```python
from build123d import *

# Parameters (mm, degrees)
F0_W     = 100
F0_H     = 100
F1_DEPTH = 100
F2_R     = 10
F3_R     = 15
F4_DEPTH = 100.001
F5_R     = 6
F6_DEPTH = 36.2532730151
F7_W     = 150
F7_H     = 100
F8_DEPTH = 25
F9_R     = 5
F11_D    = 10


with BuildPart() as f1:
    # F0 (on Front) → F1 (new body)
    with BuildSketch(Plane.XZ):
        Rectangle(F0_W, F0_H)
    extrude(amount=F1_DEPTH)

    # F2
    f2_edges = [f1.edges().sort_by_distance(p)[0] for p in [
        (50, -100, 0),
        (-50, -100, 0),
    ]]
    fillet(f2_edges, radius=F2_R)

    # F3 (on face) → F4 (cut, through all)
    with BuildSketch(Plane.XY.offset(50)):
        with Locations((0, -50)):
            Circle(F3_R)
    extrude(amount=-F4_DEPTH, mode=Mode.SUBTRACT)

    # F5 (on face) → F6 (cut, through all)
    with BuildSketch(Plane.XZ.offset(100)):
        Circle(F5_R)
    extrude(amount=-F6_DEPTH, mode=Mode.SUBTRACT)

    # F7 (on Front) → F8 (join)
    with BuildSketch(Plane.XZ):
        Rectangle(F7_W, F7_H)
    extrude(amount=-F8_DEPTH)

    # F9
    f9_edges = [f1.edges().sort_by_distance(p)[0] for p in [
        (50, 0, 0),
        (-50, 0, 0),
    ]]
    fillet(f9_edges, radius=F9_R)

    # F11 (through all)
    with Locations(Plane.XZ):
        with Locations((-65, 25), (-65, -25), (65, 25), (65, -25)):
            Hole(F11_D / 2)


solid = f1.part
```
Input: part model. Units: mm. Frame: model coordinates. A direction names the side the tool comes from. Give positions to 0.01 mm unless a question says otherwise; leave off trailing zeros. Order: outer loops, then holes, each group sorted by start corner. A loop starts at its lowest first (then second) coordinate and runs counter-clockwise, first axis right, second up. Notation, with made-up numbers: (27.5, 63) - (72.5, 63) arc R11 ccw to (72.5, 70) - close; hole circle Ø6 at (77.25, 33). An arc over 180 degrees is marked (long way). One line per item, written item: value.
1. Cut plane A-A, the plane z = 25. Output: boundary loops of the cut face in (x, y), and give its area (3 significant figures).
Determined:
outline: (-75, 0) - (-70, 0) - (-70, 25) - (-75, 25) - close; (-60, 0) - (-55, 0) arc R5 cw to (-50, -5) - (-50, -90) arc R10 ccw to (-40, -100) - (40, -100) arc R10 ccw to (50, -90) - (50, -5) arc R5 cw to (55, 0) - (60, 0) - (60, 25) - (-60, 25) - close; (70, 0) - (75, 0) - (75, 25) - (70, 25) - close; hole circle Ø30 at (0, -50)
area: 12,500 mm2
2. Cut plane D-D, the plane z = 0. Output: boundary loops of the cut face in (x, y), and give its area (3 significant figures).
Determined:
outline: (-75, 0) - (-55, 0) arc R5 cw to (-50, -5) - (-50, -90) arc R10 ccw to (-40, -100) - (-6, -100) - (-6, -63.75) arc R15 cw (long way) to (6, -63.75) - (6, -100) - (40, -100) arc R10 ccw to (50, -90) - (50, -5) arc R5 cw to (55, 0) - (75, 0) - (75, 25) - (-75, 25) - close
area: 12,600 mm2
3. Pin query (flat end, axial travel): pin 1 Ø6 at (y, z) = (-27, 1.5) entering from +X; pin 2 Ø12 at (x, z) = (48, -5) entering from -Y; pin 3 Ø10 at (x, z) = (-62.5, 24) entering from -Y; pin 4 Ø10 at (x, z) = (42.5, -29) entering from -Y. Return the tip coordinate at first contact, or that it passes through.
Determined:
pin 1: x = 50
pin 2: y = -99.8
pin 3: y = 0
pin 4: y = -100
4. Line query: probe 1 along Z at (x, y) = (-65, 15.5); probe 2 along X at (y, z) = (-82, 0); probe 3 along X at (y, z) = (-85, 11). Output: solid intervals per line, ascending.
Determined:
probe 1: -50 to -30, -20 to 20, 30 to 50
probe 2: -50 to -6, 6 to 50
probe 3: -50 to 50
5. Cut plane C-C, the plane y = -59. Output: boundary loops of the cut face in (x, z), and give its area (3 significant figures).
Determined:
outline: (-50, -50) - (-12, -50) - (-12, 50) - (-50, 50) - close; (12, -50) - (50, -50) - (50, 50) - (12, 50) - close
area: 7,600 mm2
6. Cut plane B-B, the plane x = -65. Output: boundary loops of the cut face in (y, z), and give its area (3 significant figures).
Determined:
outline: (0, -50) - (25, -50) - (25, -30) - (0, -30) - close; (0, -20) - (25, -20) - (25, 20) - (0, 20) - close; (0, 30) - (25, 30) - (25, 50) - (0, 50) - close
area: 2,000 mm2
7. Reachability of faces 4 (the face through (-65, 0, 1)), 5 (the face through (66.08, 12.68, 20.12)), 6 (the face through (65, 0, 1)) from +Z, -Z, +X, -X, +Y, -Y: full face, straight path, thin tool, end or side. Return the list, or none.
Determined:
face 4: +Z, -Z, -X, -Y
face 5: +Y, -Y
face 6: +Z, -Z, +X, -Y
8. Draft query along Z for faces 1 (the face through (-6, -82, 0)), 2 (the face through (75, 12, -1)), 3 (the face through (-1, -24, 50)). Return one class per face: released by +Z, released by -Z, zero draft, split by the parting line, or undercut.
Determined:
face 1: undercut
face 2: zero draft
face 3: released by +Z
